Autodesk Fusion 360 part; units mm, degrees
sketch "Sketch1" plane through (0, 0, 0) normal (0, 1, 0) x (1, 0, 0)
  line L0 (-20, -35) -> (20, -35)
  line L1 (20, -35) -> (20, 35)
  line L2 (20, 35) -> (-20, 35)
  line L3 (-20, 35) -> (-20, -35)
  line L4 (-14.65, -4.5) -> (-12.65, -4.5)
  line L5 (-12.65, -4.5) -> (-12.65, 4.5)
  line L6 (-12.65, 4.5) -> (-14.65, 4.5)
  line L7 (-14.65, 4.5) -> (-14.65, -4.5)
  line L8 (12.65, -4.5) -> (14.65, -4.5)
  line L9 (14.65, -4.5) -> (14.65, 4.5)
  line L10 (14.65, 4.5) -> (12.65, 4.5)
  line L11 (12.65, 4.5) -> (12.65, -4.5)
  line L12 (-12.65, -4.5) -> (-11.65, -4.5)
  line L13 (-11.65, -4.5) -> (-11.65, 4.5)
  line L14 (-11.65, 4.5) -> (-12.65, 4.5)
  line L15 (-12.65, 4.5) -> (-12.65, -4.5)
  line L16 (12.65, -4.5) -> (11.65, -4.5)
  line L17 (11.65, -4.5) -> (11.65, 4.5)
  line L18 (11.65, 4.5) -> (12.65, 4.5)
  line L19 (12.65, 4.5) -> (12.65, -4.5)
  circle A0 centre (0, 0) radius 5
  line L20 (14, 16.5) -> (14, 25.5)
  line L21 (15, 16.5) -> (14, 16.5)
  line L22 (17, 16.5) -> (17, 25.5)
  line L23 (15, 25.5) -> (15, 16.5)
  line L24 (15, 16.5) -> (17, 16.5)
  line L25 (15, 25.5) -> (15, 16.5)
  line L26 (15, -19.5) -> (15, -28.5)
  line L27 (15, -19.5) -> (15, -28.5)
  line L28 (15, -28.5) -> (17, -28.5)
  line L29 (14, -28.5) -> (14, -19.5)
  line L30 (15, -28.5) -> (14, -28.5)
  line L31 (17, -28.5) -> (17, -19.5)
  line L32 (-15, -28.5) -> (-15, -19.5)
  line L33 (-17, -19.5) -> (-17, -28.5)
  line L34 (-15, -28.5) -> (-14, -28.5)
  line L35 (-14, -28.5) -> (-14, -19.5)
  line L36 (-15, -19.5) -> (-17, -19.5)
  line L37 (-15, -19.5) -> (-15, -28.5)
  line L38 (-14, -19.5) -> (-15, -19.5)
  line L39 (-17, -28.5) -> (-15, -28.5)
  line L40 (-15, 16.5) -> (-15, 25.5)
  line L41 (-17, 25.5) -> (-17, 16.5)
  line L42 (-15, 16.5) -> (-14, 16.5)
  line L43 (-14, 16.5) -> (-14, 25.5)
  line L44 (-15, 25.5) -> (-17, 25.5)
  line L45 (-15, 25.5) -> (-15, 16.5)
  line L46 (-14, 25.5) -> (-15, 25.5)
  line L47 (-17, 16.5) -> (-15, 16.5)
  line L48 (17, 25.5) -> (14, 25.5)
  line L49 (17, -19.5) -> (14, -19.5)
  line L50 (12.65, 1.5) -> (14.65, 1.5)
  line L51 (-14.65, 1.5) -> (-12.65, 1.5)
  line L52 (-10, -18) -> (10, -18)
  line L53 (10, -18) -> (10, 7)
  line L54 (10, 7) -> (-10, 7)
  line L55 (-10, 7) -> (-10, -18)
  line L56 (16.5, 1.5) -> (10.5, 1.5)
  line L57 (10.5, 1.5) -> (10.5, 6.5)
  line L58 (10.5, 6.5) -> (16.5, 6.5)
  line L59 (16.5, 6.5) -> (16.5, 1.5)
  line L60 (-10.5, 1.5) -> (-16.5, 1.5)
  line L61 (-16.5, 1.5) -> (-16.5, 6.5)
  line L62 (-16.5, 6.5) -> (-10.5, 6.5)
  line L63 (-10.5, 6.5) -> (-10.5, 1.5)
  dimension "d1" = 40
  dimension "d2" = 70
  dimension "d3" = 20
  dimension "d4" = 35
  dimension "d5" = 9
  dimension "d6" = 2
  dimension "d7" = 4.5
  dimension "d8" = 12.65
  dimension "d9" = 2
  dimension "d10" = 9
  dimension "d11" = 12.65
  dimension "d12" = 4.5
  dimension "d13" = 1
  dimension "d14" = 9
  dimension "d15" = 1
  dimension "d16" = 9
  dimension "d17" = 10
  dimension "d18" = 2
  dimension "d19" = 9
  dimension "d20" = 1
  dimension "d21" = 9
  dimension "d22" = 2
  dimension "d23" = 9
  dimension "d24" = 1
  dimension "d25" = 9
  dimension "d26" = 9
  dimension "d27" = 2
  dimension "d28" = 1
  dimension "d29" = 9
  dimension "d30" = 9
  dimension "d31" = 2
  dimension "d32" = 1
  dimension "d33" = 9
  dimension "d40" = 3
  dimension "d41" = 3
  dimension "d58" = 20
  dimension "d59" = 25
  dimension "d60" = 10
  dimension "d61" = 18
  dimension "d64" = 6
  dimension "d65" = 5
  dimension "d66" = 2.15
  dimension "d67" = 2.15
  dimension "d79" = 3
  dimension "d80" = 3
  dimension "d81" = 3
  dimension "d82" = 3
extrude "Extrude1" add sketch "Sketch1" along normal blind 3 contours L0 L1 L2 L3 | L4 L5 L7 L15 L51 L60 | L5 L12 L13 L15 L60 | L6 L7 L13 L14 L60 L61 L62 L63 | L5 L6 L7 L15 L51 L60 | L5 L13 L14 L15 L60 | L8 L9 L11 L19 L50 L56 | L11 L16 L17 L19 L56 | L11 L17 L18 L19 L56 | L9 L10 L11 L19 L50 L56 | L9 L10 L17 L18 L56 L57 L58 L59 | A0 | L20 L21 L23 L25 L48 | L22 L23 L24 L25 L48 | L26 L27 L28 L31 L49 | L26 L27 L29 L30 L49 | L32 L33 L36 L37 L39 | L32 L34 L35 L37 L38 | L40 L41 L44 L45 L47 | L40 L42 L43 L45 L46 | L52 L53 L54 L55
extrude "Extrude2" add sketch "Sketch1" against normal blind 14 contours L6 L7 L13 L14 L60 L61 L62 L63 | L5 L6 L7 L15 L51 L60 | L5 L13 L14 L15 L60 | L11 L17 L18 L19 L56 | L9 L10 L11 L19 L50 L56 | L9 L10 L17 L18 L56 L57 L58 L59
extrude "Extrude4" add sketch "Sketch1" along normal blind 20 contours L20 L21 L23 L25 L48 | L22 L23 L24 L25 L48 | L26 L27 L28 L31 L49 | L26 L27 L29 L30 L49 | L32 L33 L36 L37 L39 | L32 L34 L35 L37 L38 | L40 L41 L44 L45 L47 | L40 L42 L43 L45 L46
extrude "Extrude5" cut sketch "Sketch1" along normal blind 19 contours L20 L21 L23 L25 L48 | L26 L27 L29 L30 L49 | L32 L34 L35 L37 L38 | L40 L42 L43 L45 L46
extrude "Extrude6" add sketch "Sketch1" along normal blind 14 contours L20 L21 L23 L25 L48 | L26 L27 L29 L30 L49 | L32 L34 L35 L37 L38 | L40 L42 L43 L45 L46
chamfer "Chamfer3" distance 2 angle 45 12 edges at (-15.5, 3, -16.5) (-17, 3, 24) (-17, 3, -21) (-15.5, 3, -25.5) (15.5, 3, -25.5) (17, 3, -21) (15.5, 3, -16.5) (15.5, 3, 19.5) (17, 3, 24) (15.5, 3, 28.5) (-15.5, 3, 28.5) (-15.5, 3, 19.5)
extrude "Extrude7" add sketch "Sketch1" against normal blind 4 contours A0 | L52 L53 L54 L55
sketch "Sketch2" plane through (0, 0, -1.5) normal (0, 0, 1) x (-1, 0, 0)
  line L0 (10.5, 0) -> (16.5, 0)
  line L1 (16.5, 0) -> (16.5, 14)
  line L2 (16.5, 14) -> (10.5, 14)
  line L3 (10.5, 14) -> (10.5, 0)
  circle A0 centre (13.5, 10.39) radius 1
  circle A1 centre (-13.5, 10.39) radius 1
  line L4 (-10.5, 0) -> (-10.5, 14)
  line L5 (20, 0) -> (-20, 0)
  dimension "d68" = 2
  dimension "d70" = 10.39
  dimension "d71" = 3
  dimension "d72" = 2
  dimension "d73" = 3
  dimension "d74" = 10.39
extrude "Extrude8" cut sketch "Sketch2" against normal blind 9 contours A0 | A1
chamfer "Chamfer4" distance 3 angle 45 6 edges at (16.5, 0, -4) (13.5, 0, -1.5) (13.5, 0, -6.5) (-13.5, 0, -6.5) (-16.5, 0, -4) (-13.5, 0, -1.5)
move_face "OffsetFaces1" offset -0.5 2 faces at (10.5, -6.6667, -4.8333) (-10.5, -6.6667, -3.1667)
Work out the finished part from the listing and answer in its coordinate system (mm). A direction names the side the tool comes from. Give positions to 0.01 mm unless a question says otherwise; leave off trailing zeros. Loops run counter-clockwise (first coordinate to the right, second up) from the corner with the lowest first, then second, coordinate; pieces in that order, holes last. Notation, with made-up numbers: (1, -4.75) -> (42, -4.75) arc R27 ccw to (42, 28.25) -> close; hole circle Ø3 at (46.5, 34). An arc over 180 degrees is marked (long way). Use CSV: the item, a comma, the result in double quotes.
1. The mould has two halves that part along X. Classify faces 6 (the flat face through (-16, 4, -15.5)), 7 (the flat face through (10, -2, 6)), 8 (the flat face through (16.5, -8, -4)): +X half, -X half, draft (parallel to the pull), parting line (faces both ways), or undercut.
Found:
face 6,"draft"
face 7,"undercut"
face 8,"+X half"
2. The part is cut by section C-C (z = 22). Write down the section's boundary in (x, y).
Found:
outline,"(-20, 0) -> (20, 0) -> (20, 3) -> (19, 3) -> (17, 5) -> (17, 20) -> (14, 20) -> (14, 19) -> (15, 19) -> (15, 14) -> (14, 14) -> (14, 3) -> (-14, 3) -> (-14, 14) -> (-15, 14) -> (-15, 19) -> (-14, 19) -> (-14, 20) -> (-17, 20) -> (-17, 5) -> (-19, 3) -> (-20, 3) -> close"
3. The part is cut by section A-A (y = -10.39). Write down the section's boundary in (x, z).
Found:
outline,"(-16.5, -6.5) -> (-14.5, -6.5) -> (-14.5, -1.5) -> (-16.5, -1.5) -> close; (-12.5, -6.5) -> (-11, -6.5) -> (-11, -1.5) -> (-12.5, -1.5) -> close; (11, -6.5) -> (12.5, -6.5) -> (12.5, -1.5) -> (11, -1.5) -> close; (14.5, -6.5) -> (16.5, -6.5) -> (16.5, -1.5) -> (14.5, -1.5) -> close"
4. The part is cut by section D-D (y = 13). Write down the section's boundary in (x, z), then the cut area to 3 significant figures.
Found:
outline,"(-17, -25.5) -> (-14, -25.5) -> (-14, -16.5) -> (-17, -16.5) -> close; (-17, 19.5) -> (-14, 19.5) -> (-14, 28.5) -> (-17, 28.5) -> close; (14, -25.5) -> (17, -25.5) -> (17, -16.5) -> (14, -16.5) -> close; (14, 19.5) -> (17, 19.5) -> (17, 28.5) -> (14, 28.5) -> close"
area,"108 mm^2"
5. Straight lines are drawn through the part: line 1 (X direction, y = -10.39, z = -3.75); line 2 (Y direction, x = -13.5, z = -4.55); line 3 (X direction, y = -10, z = -3). For each, find the intervals that lie inside material, in ascending order.
Found:
line 1,"-16.5 to -14.5, -12.5 to -11, 11 to 12.5, 14.5 to 16.5"
line 2,"-14 to -11.39, -9.39 to 3"
line 3,"-16.5 to -14.42, -12.58 to -11, 11 to 12.58, 14.42 to 16.5"
6. The part is cut by section B-B (x = -3). Write down the section's boundary in (y, z), then the cut area to 3 significant figures.
Found:
outline,"(-4, -7) -> (0, -7) -> (0, -35) -> (3, -35) -> (3, 35) -> (0, 35) -> (0, 18) -> (-4, 18) -> close"
area,"310 mm^2"
7. A tool of negligible diameter and unlimited length cuts with its end or side. For faces 1 (the flat face through (11, -7, -4)), 2 (the flat face through (17, 12, -21)), 3 (the flat face through (0, -2, -7)), 4 (the flat face through (16, 12, 19.5)), 5 (the flat face through (0, 0, -8)), from which of +Z, -Z, +X, -X, +Y, -Y can it reach the whole face along a straight path? Write none if from no direction.
Found:
face 1,"+Z, -Z, -Y"
face 2,"+Z, -Z, +X, +Y"
face 3,"-Z, -Y"
face 4,"+X, -X, +Y"
face 5,"-Y"
8. Flat-ended cylindrical pins translate along their axes: pin 1 Ø0.8 at (x, z) = (-14.5, -22.5) entering from -Y; pin 2 Ø10 at (y, z) = (9, 24) entering from -X; pin 3 Ø3.5 at (x, y) = (-15, 13.5) entering from +Z; pin 4 Ø3 at (y, z) = (-1, 23) entering from -X. Find the tip coordinate at first contact, or state that the pin passes through.
Found:
pin 1,"y = 0"
pin 2,"x = -18"
pin 3,"z = 28.5"
pin 4,"x = -20"
